Check sheet for the drawn part. Datum: minimum x, y, z corner. Units: mm. A direction names the side the tool comes from. Coordinates: 2 decimals unless noted, no trailing zeros. Loops run counter-clockwise (first coordinate to the right, second up) from the corner with the lowest first, then second, coordinate; pieces in that order, holes last.
Q1. Material ranges on probe 1 along Z at (x, y) = (2.2, 2.5); probe 2 along Y at (x, z) = (2.85, 2.7); probe 3 along Y at (x, z) = (1.75, 1.85), recorded low to high.
Q2. Sectioned sample at A-A (x = 2.75). Enter the section's corners in (y, z), then the cut area to 3 significant figures.
Q3. Mould release check, pull along Y, two halves, no side actions. Record for the marked faces 3, 4 and 5: +Y half, -Y half, draft (parallel to the pull), parting line (faces both ways), or undercut.
Q4. Sectioned sample at C-C (y = 11.75). Enter the section's corners in (x, z), then the cut area to 3 significant figures.
Q5. Sectioned sample at D-D (z = 2). Count the separate pieces of the cut face and the enclosed holes in it, then the cut area to 3 significant figures.
Q6. Access from +Z, -Z, +X, -X, +Y, -Y to the whole of each face (thin tool, end or side, straight path). Record for the marked faces 1 and 2.
Q7. Sectioned sample at B-B (y = 6). Enter the section's corners in (x, z).
Q8. Go/stop test with flat-tipped pins: P1, Ø0.8, axis at x = 1, z = 4.5, coming from the +Y side; P2, Ø0.5, axis at x = 2, z = 4.5, coming from the -Y side. Record where each tip stops, or that it passes through.
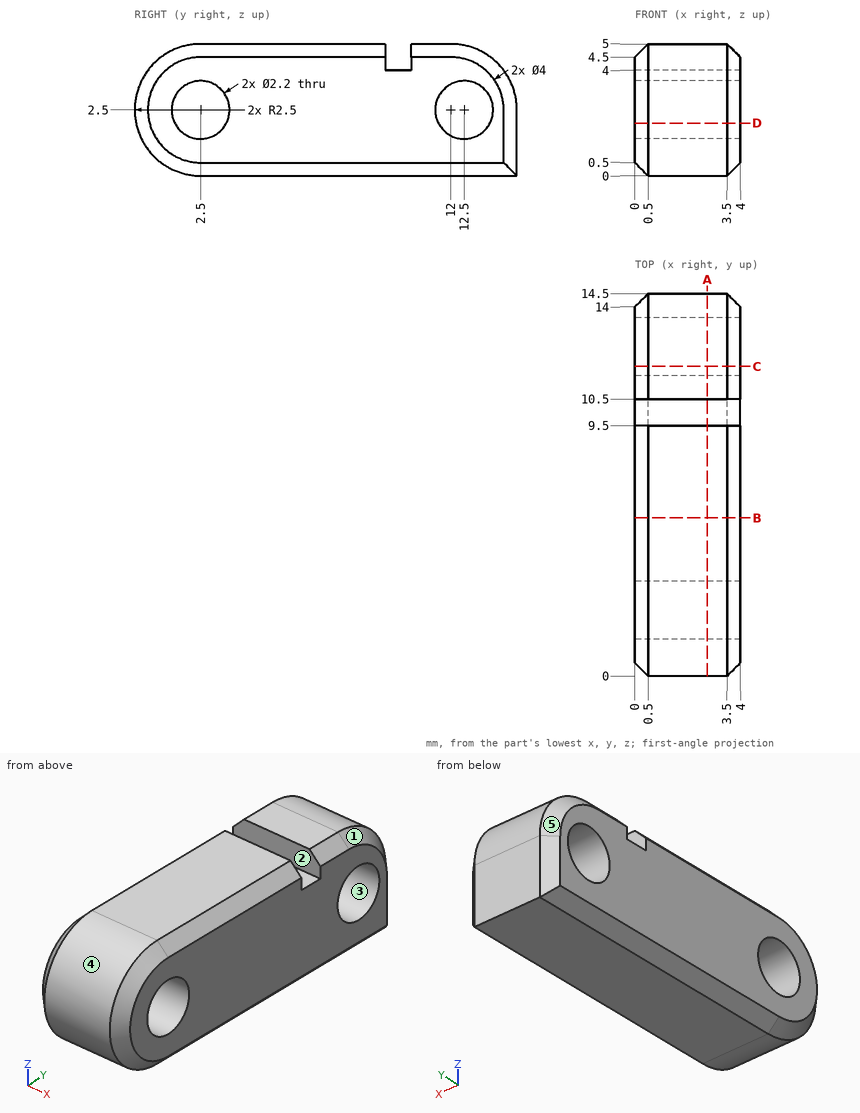
Geometry check:
1. probe 1: z = 0 to 1.4, 3.6 to 5
1. probe 2: y = 0.01 to 1.42, 3.58 to 11.42, 13.58 to 14.49
1. probe 3: y = 0.09 to 1.61, 3.39 to 11.61, 13.39 to 14.5
2. outline: (2.5, 0) - (14.5, 0) - (14.5, 2.5) arc R2.5 ccw to (12, 5) - (10.5, 5) - (10.5, 4) - (9.5, 4) - (9.5, 5) - (2.5, 5) arc R2.5 ccw to start; hole circle Ø2.2 at (2.5, 2.5); hole circle Ø2.2 at (12.5, 2.5)
2. area: 59.9 mm2
3. face 3: undercut
3. face 4: -Y half
3. face 5: +Y half
4. outline: (0, 0.5) - (0.5, 0) - (3.5, 0) - (4, 0.5) - (4, 1.7) - (0, 1.7) - close; (0, 3.3) - (4, 3.3) - (4, 4.5) - (3.5, 5) - (0.5, 5) - (0, 4.5) - close
4. area: 13.1 mm2
5. separate pieces: 3
5. enclosed holes: 0
5. area: 41.6 mm2
6. face 1: +Z, +X, +Y
6. face 2: +Z, +X, -X
7. outline: (0, 0.5) - (0.5, 0) - (3.5, 0) - (4, 0.5) - (4, 4.5) - (3.5, 5) - (0.5, 5) - (0, 4.5) - close
8. P1: stops at y = 13.92
8. P2: stops at y = 0.71
